```python
from build123d import *

# Parameters (mm, degrees)
SKETCH2_W                            = 101.6
SKETCH2_H                            = 127
BOSS_EXTRUDE1_DEPTH                  = 76.2
SHELL1_T                             = -6.35
F_11_64_0_17188_DIAMETER_HOLE1_D     = 4.365752
F_11_64_0_17188_DIAMETER_HOLE1_DEPTH = 25.4
F_11_64_0_17188_DIAMETER_HOLE1_TIP   = 1.311604225
SKETCH4_R                            = 5.715
CUT_EXTRUDE2_DEPTH                   = 112.44204772
SKETCH6_W                            = 19.05
SKETCH6_H                            = 28.575
SKETCH6_R                            = 5.715
BOSS_EXTRUDE2_DEPTH                  = 25.4
F_11_64_0_17188_DIAMETER_HOLE2_D     = 4.365752
F_11_64_0_17188_DIAMETER_HOLE2_DEPTH = 127
F_11_64_0_17188_DIAMETER_HOLE2_TIP   = 1.311604225
CUT_EXTRUDE3_REACH                   = 143.99
SKETCH9_R                            = 3.81
SKETCH10_W                           = 25.4
SKETCH10_H                           = 44.45
CUT_EXTRUDE5_DEPTH                   = 108.200338152
SKETCH11_R                           = 3.175
CUT_EXTRUDE6_DEPTH                   = 157.576115675
CUT_EXTRUDE7_REACH                   = 143.99
SKETCH13_R                           = 2.54
SKETCH14_W                           = 41.275
SKETCH14_H                           = 41.275
CUT_EXTRUDE8_DEPTH                   = 2.032


with BuildPart() as part:
    # Sketch2 → Boss-Extrude1 (new body)
    with BuildSketch(Plane(origin=(0, 0, 0), x_dir=(1, 0, 0), z_dir=(0, 1, 0))):
        Rectangle(SKETCH2_W, SKETCH2_H)
    extrude(amount=BOSS_EXTRUDE1_DEPTH)

    # Shell1
    shell1_openings = [part.faces().sort_by_distance(p)[0] for p in [
        (0, 0, 0),
    ]]
    offset(amount=SHELL1_T, openings=shell1_openings, kind=Kind.INTERSECTION)

    # 11/64 (0.17188) Diameter Hole1
    with Locations(Plane(origin=(-19.05, 76.2, -44.45), x_dir=(0, 0, 1), z_dir=(0, 1, 0))):
        with Locations((0, 0), (0, 38.1), (88.9, 0), (88.9, 38.1)):
            Hole(F_11_64_0_17188_DIAMETER_HOLE1_D / 2, depth=F_11_64_0_17188_DIAMETER_HOLE1_DEPTH)
            with Locations((0, 0, -(F_11_64_0_17188_DIAMETER_HOLE1_DEPTH + F_11_64_0_17188_DIAMETER_HOLE1_TIP / 2))):  # 118° drill point
                Cone(0, F_11_64_0_17188_DIAMETER_HOLE1_D / 2, F_11_64_0_17188_DIAMETER_HOLE1_TIP, mode=Mode.SUBTRACT)

    # Sketch4 → Cut-Extrude2 (cut, through all)
    with BuildSketch(Plane(origin=(0, 76.2, 0), x_dir=(1, 0, 0), z_dir=(0, 1, 0))):
        with Locations(Location((0, 44.45, 0), (0, 0, 270))):
            Circle(SKETCH4_R)
        with Locations(Location((0, -44.45, 0), (0, 0, 270))):
            Circle(SKETCH4_R)
    extrude(amount=-CUT_EXTRUDE2_DEPTH, mode=Mode.SUBTRACT)

    # Sketch6 → Boss-Extrude2 (add)
    # profile 1 of 2: a face of its own
    with BuildSketch(Plane.XZ.offset(-69.85)):
        with Locations((0, 42.8625)):
            Rectangle(SKETCH6_W, SKETCH6_H)
        with Locations(Location((0, 44.45, 0), (0, 0, 90))):
            Circle(SKETCH6_R, mode=Mode.SUBTRACT)
    # profile 2 of 2: a face of its own
    with BuildSketch(Plane.XZ.offset(-69.85)):
        with Locations((0, -42.8625)):
            Rectangle(SKETCH6_W, SKETCH6_H)
        with Locations(Location((0, -44.45, 0), (0, 0, 90))):
            Circle(SKETCH6_R, mode=Mode.SUBTRACT)
    extrude(amount=BOSS_EXTRUDE2_DEPTH)

    # 11/64 (0.17188) Diameter Hole2
    with Locations(Plane(origin=(-50.8, 51.816, -23.622), x_dir=(0, 0, -1), z_dir=(-1, 0, 0))):
        with Locations((0, 0), (0, 47.244), (-47.244, 0), (-47.244, 47.244)):
            Hole(F_11_64_0_17188_DIAMETER_HOLE2_D / 2, depth=F_11_64_0_17188_DIAMETER_HOLE2_DEPTH)
            with Locations((0, 0, -(F_11_64_0_17188_DIAMETER_HOLE2_DEPTH + F_11_64_0_17188_DIAMETER_HOLE2_TIP / 2))):  # 118° drill point
                Cone(0, F_11_64_0_17188_DIAMETER_HOLE2_D / 2, F_11_64_0_17188_DIAMETER_HOLE2_TIP, mode=Mode.SUBTRACT)

    # Sketch9 → Cut-Extrude3 (cut, up to next)
    with BuildSketch(Plane.ZY.offset(50.8), mode=Mode.PRIVATE) as cut_extrude3_sk1:
        with Locations((0, 28.194)):
            Circle(SKETCH9_R)
    cut_extrude3_tool1 = extrude(cut_extrude3_sk1.sketch, amount=-CUT_EXTRUDE3_REACH, mode=Mode.PRIVATE) & part.part
    add(cut_extrude3_tool1.solids().sort_by_distance((-50.8, 28.194, 0))[0], mode=Mode.SUBTRACT)

    # Sketch10 → Cut-Extrude5 (cut, through all)
    with BuildSketch(Plane(origin=(0, 69.85, 0), x_dir=(-1, 0, 0), z_dir=(0, -1, 0))):
        with Locations((31.75, 0)):
            Rectangle(SKETCH10_W, SKETCH10_H)
        with Locations((-31.75, 0)):
            Rectangle(SKETCH10_W, SKETCH10_H)
    extrude(amount=-CUT_EXTRUDE5_DEPTH, mode=Mode.SUBTRACT)

    # Sketch11 → Cut-Extrude6 (cut, through all)
    with BuildSketch(Plane.XY.offset(63.5)):
        with Locations((-31.75, 38.1)):
            Circle(SKETCH11_R)
        with Locations((31.75, 38.1)):
            Circle(SKETCH11_R)
    extrude(amount=-CUT_EXTRUDE6_DEPTH, mode=Mode.SUBTRACT)

    # Sketch13 → Cut-Extrude7 (cut, up to next)
    with BuildSketch(Plane(origin=(50.8, 0, 0), x_dir=(0, 0, -1), z_dir=(1, 0, 0)), mode=Mode.PRIVATE) as cut_extrude7_sk1:
        with Locations((0, 28.194)):
            Circle(SKETCH13_R)
    cut_extrude7_tool1 = extrude(cut_extrude7_sk1.sketch, amount=-CUT_EXTRUDE7_REACH, mode=Mode.PRIVATE) & part.part
    add(cut_extrude7_tool1.solids().sort_by_distance((50.8, 28.194, 0))[0], mode=Mode.SUBTRACT)

    # Sketch14 → Cut-Extrude8 (cut)
    with BuildSketch(Plane.ZY.offset(50.8)):
        with Locations((0, 28.194)):
            Rectangle(SKETCH14_W, SKETCH14_H)
    extrude(amount=-CUT_EXTRUDE8_DEPTH, mode=Mode.SUBTRACT)


solid = part.part
```
Work out the finished part from the listing and answer in its coordinate system (mm). A direction names the side the tool comes from. Give positions to 0.01 mm unless a question says otherwise; leave off trailing zeros. Order: outer loops, then holes, each group sorted by start corner. A loop starts at its lowest first (then second) coordinate and runs counter-clockwise, first axis right, second up. Notation, with made-up numbers: (1, -31.75) - (25, -31.75) arc R19 cw to (25, -25.75) - close; hole circle Ø5 at (5.25, 79). An arc over 180 degrees is marked (long way). One line per item, written item: value. Start each with the question number.
1. Which of the six approach directions +Z, -Z, +X, -X, +Y, -Y give full straight-line access (tool end or side, diameter ignored) to faces 1 (the face through (0, 57, 28.575)), 2 (the face through (-48.768, 24, 0)), 3 (the face through (-19.05, 73, 0))?
2. Each of these flat-tipped pins is pushed along its axis until it touches: pin 1 Ø5.5 at (x, z) = (19.05, 44.45) entering from -Y; pin 2 Ø5 at (x, z) = (35.5, 50.5) entering from -Y; pin 3 Ø13 at (x, z) = (0, -44.45) entering from -Y. Where does it stop, or does it pass through?
3. Section A-A, the plane x = 31.75 is taken. Write down the section's boundary in (y, z) (3 decimals).
4. Consider line 1 (X direction, y = 54.5, z = 57) (3 decimals); line 2 (Z direction, x = 17.5, y = 9); line 3 (X direction, y = 31, z = -17.5). Determine where each line is inside the solid, lowest interval first.
5. For a pull along Z with two mould halves and no side action, classify faces 4 (the face through (-9.525, 57, 43)), 5 (the face through (-1, 38, 63.5)), 6 (the face through (-34.92, 38.24, 60.37)), 7 (the face through (-47.58, 52.65, 25.64)) as released by +Z, released by -Z, zero draft, split by the parting line, or undercut.
6. Section B-B, the plane z = 7 is taken. Write down the section's boundary in (x, y), then the cut area to 3 significant figures.
7. Section D-D, the plane y = 59 is taken. Write down the section's boundary in (x, z) (3 decimals), then the cut area to 3 significant figures.
8. Section C-C, the plane x = 0 is taken. Write down the section's boundary in (y, z) (3 decimals), then the cut area to 3 significant figures.
Filled sheet:
1. face 1: -Y
1. face 2: -X
1. face 3: +Y, -Y
2. pin 1: y = 69.85
2. pin 2: y = 69.85
2. pin 3: y = 44.45
3. outline: (0, -63.5) - (34.925, -63.5) - (34.925, -57.15) - (0, -57.15) - close; (0, 57.15) - (34.925, 57.15) - (34.925, 63.5) - (0, 63.5) - close; (41.275, -63.5) - (76.2, -63.5) - (76.2, -22.225) - (69.85, -22.225) - (69.85, -57.15) - (41.275, -57.15) - close; (41.275, 57.15) - (69.85, 57.15) - (69.85, 22.225) - (76.2, 22.225) - (76.2, 63.5) - (41.275, 63.5) - close
4. line 1: -50.8 to -44.45, -9.525 to 9.525, 44.45 to 50.8
4. line 2: -63.5 to -57.15, 57.15 to 63.5
4. line 3: -48.77 to -44.45, 44.45 to 50.8
5. face 4: undercut
5. face 5: released by +Z
5. face 6: zero draft
5. face 7: undercut
6. outline: (-50.8, 0) - (-44.45, 0) - (-44.45, 76.2) - (-50.8, 76.2) - (-50.8, 48.83) - (-48.77, 48.83) - (-48.77, 7.56) - (-50.8, 7.56) - close; (-19.05, 69.85) - (19.05, 69.85) - (19.05, 76.2) - (-19.05, 76.2) - close; (44.45, 0) - (50.8, 0) - (50.8, 76.2) - (44.45, 76.2) - close
6. area: 1,130 mm²
7. outline: (-50.8, -63.5) - (50.8, -63.5) - (50.8, 63.5) - (-50.8, 63.5) - close; hole (-44.45, -57.15) - (-9.525, -57.15) - (-9.525, -28.575) - (9.525, -28.575) - (9.525, -57.15) - (44.45, -57.15) - (44.45, 57.15) - (9.525, 57.15) - (9.525, 28.575) - (-9.525, 28.575) - (-9.525, 57.15) - (-44.45, 57.15) - close; hole circle Ø11.43 at (0, -44.45); hole circle Ø11.43 at (0, 44.45)
7. area: 3,630 mm²
8. outline: (0, -63.5) - (76.2, -63.5) - (76.2, -50.165) - (44.45, -50.165) - (44.45, -57.15) - (0, -57.15) - close; (0, 57.15) - (44.45, 57.15) - (44.45, 50.165) - (76.2, 50.165) - (76.2, 63.5) - (0, 63.5) - close; (44.45, -38.735) - (76.2, -38.735) - (76.2, 38.735) - (44.45, 38.735) - (44.45, 28.575) - (69.85, 28.575) - (69.85, -28.575) - (44.45, -28.575) - close
8. area: 2,420 mm²
